Check sheet for the modelled part. Datum: model origin and axes. Units: mm. Give positions to 0.01 mm unless a question says otherwise; leave off trailing zeros. Write each loop counter-clockwise with the first axis right and the second up, starting at its lowest first coordinate (ties: lowest second). Pieces come first, ordered by that corner, then holes.
from build123d import *
from build123d.topology import SkipClean

# Parameters (mm, degrees)
SKETCH1_R           = 7.5
SKETCH1_R_2         = 4
BOSS_EXTRUDE1_DEPTH = 5
BOSS_EXTRUDE2_START = 1.1
SKETCH2_R           = 7
SKETCH2_R_2         = 4
BOSS_EXTRUDE2_DEPTH = 1.1
BOSS_EXTRUDE3_START = 32.8
SKETCH3_R           = 7.5
SKETCH3_R_2         = 4
BOSS_EXTRUDE3_DEPTH = 32.8
BOSS_EXTRUDE5_START = 1.1
SKETCH5_R           = 7
SKETCH5_R_2         = 4
BOSS_EXTRUDE5_DEPTH = 1.1
BOSS_EXTRUDE6_START = 5
SKETCH6_R           = 7.5
SKETCH6_R_2         = 4
BOSS_EXTRUDE6_DEPTH = 5


with BuildPart() as part:
    # Sketch1 → Boss-Extrude1 (new body)
    with BuildSketch(Plane(origin=(0, 0, 0), x_dir=(1, 0, 0), z_dir=(0, 1, 0))):
        with Locations(Location((0, 0, 0), (0, 0, 270))):
            Circle(SKETCH1_R)
        with Locations(Location((0, 0, 0), (0, 0, 270))):
            Circle(SKETCH1_R_2, mode=Mode.SUBTRACT)
    extrude(amount=BOSS_EXTRUDE1_DEPTH)

    # Sketch2 → Boss-Extrude2 (add)
    with SkipClean():  # the faces are left unmerged after this step: merging them gives an invalid solid
        with BuildSketch(Plane.XZ.offset(BOSS_EXTRUDE2_START)):
            with Locations(Location((0, 0, 0), (0, 0, 90))):
                Circle(SKETCH2_R)
            with Locations(Location((0, 0, 0), (0, 0, 270))):
                Circle(SKETCH2_R_2, mode=Mode.SUBTRACT)
        extrude(amount=-BOSS_EXTRUDE2_DEPTH)

    # Sketch3 → Boss-Extrude3 (add)
    with SkipClean():  # the faces are left unmerged after this step: merging them gives an invalid solid
        with BuildSketch(Plane.XZ.offset(1.1).offset(BOSS_EXTRUDE3_START)):
            with Locations(Location((0, 0, 0), (0, 0, 90))):
                Circle(SKETCH3_R)
            with Locations(Location((0, 0, 0), (0, 0, 270))):
                Circle(SKETCH3_R_2, mode=Mode.SUBTRACT)
        extrude(amount=-BOSS_EXTRUDE3_DEPTH)

    # Sketch5 → Boss-Extrude5 (add)
    with SkipClean():  # the faces are left unmerged after this step: merging them gives an invalid solid
        with BuildSketch(Plane.XZ.offset(33.9).offset(BOSS_EXTRUDE5_START)):
            with Locations(Location((0, 0, 0), (0, 0, 90))):
                Circle(SKETCH5_R)
            with Locations(Location((0, 0, 0), (0, 0, 270))):
                Circle(SKETCH5_R_2, mode=Mode.SUBTRACT)
        extrude(amount=-BOSS_EXTRUDE5_DEPTH)

    # Sketch6 → Boss-Extrude6 (add)
    with SkipClean():  # the faces are left unmerged after this step: merging them gives an invalid solid
        with BuildSketch(Plane.XZ.offset(35).offset(BOSS_EXTRUDE6_START)):
            with Locations(Location((0, 0, 0), (0, 0, 90))):
                Circle(SKETCH6_R)
            with Locations(Location((0, 0, 0), (0, 0, 270))):
                Circle(SKETCH6_R_2, mode=Mode.SUBTRACT)
        extrude(amount=-BOSS_EXTRUDE6_DEPTH)


solid = part.part
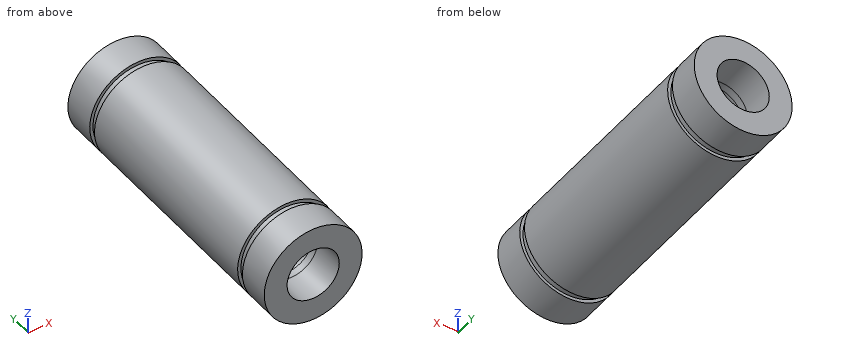
1) Sectioned sample at B-B on x = 0. Record the boundary of the cut face in (y, z), then the cut area to 3 significant figures.
2) Gauge pin test, flat ends, axial feed: pin 1 (1 mm diameter, centred on y = -30.5, z = -5.5, fed in from -X); pin 2 (5 mm diameter, centred on x = -6, y = -3.5, fed in from +Z); pin 3 (6 mm diameter, centred on x = 5.5, y = 0.5, fed in from +Z). Record the tip position at first contact, or that the pin passes through.
3) Sectioned sample at C-C on z = 5.5. Record the boundary of the cut face in (x, y).
4) Scan lines: L1, parallel to Y at x = -6.25, z = 3.5; L2, parallel to X at y = -37.15, z = 0; L3, parallel to X at y = -0.5, z = 5.75. Record each from-to range of solid material in increasing order.
5) Sectioned sample at A-A on z = 0. Record the boundary of the cut face in (x, y).
6) Sectioned sample at D-D on x = 5. Record the boundary of the cut face in (y, z).
Answers below:
1. outline: (-40, -7.5) - (-35, -7.5) - (-35, -7) - (-33.9, -7) - (-33.9, -7.5) - (-1.1, -7.5) - (-1.1, -7) - (0, -7) - (0, -7.5) - (5, -7.5) - (5, -4) - (-40, -4) - close; (-40, 4) - (5, 4) - (5, 7.5) - (0, 7.5) - (0, 7) - (-1.1, 7) - (-1.1, 7.5) - (-33.9, 7.5) - (-33.9, 7) - (-35, 7) - (-35, 7.5) - (-40, 7.5) - close
1. area: 313 mm2
2. pin 1: stops at x = -5.59
2. pin 2: stops at z = 6.63
2. pin 3: stops at z = 7.07
3. outline: (-5.1, -40) - (5.1, -40) - (5.1, -35) - (4.33, -35) - (4.33, -33.9) - (5.1, -33.9) - (5.1, -1.1) - (4.33, -1.1) - (4.33, 0) - (5.1, 0) - (5.1, 5) - (-5.1, 5) - (-5.1, 0) - (-4.33, 0) - (-4.33, -1.1) - (-5.1, -1.1) - (-5.1, -33.9) - (-4.33, -33.9) - (-4.33, -35) - (-5.1, -35) - close
4. L1: y = -40 to -35, -33.9 to -1.1, 0 to 5
4. L2: x = -7.5 to -4, 4 to 7.5
4. L3: x = -3.99 to 3.99
5. outline: (-7.5, -40) - (-4, -40) - (-4, 5) - (-7.5, 5) - (-7.5, 0) - (-7, 0) - (-7, -1.1) - (-7.5, -1.1) - (-7.5, -33.9) - (-7, -33.9) - (-7, -35) - (-7.5, -35) - close; (4, -40) - (7.5, -40) - (7.5, -35) - (7, -35) - (7, -33.9) - (7.5, -33.9) - (7.5, -1.1) - (7, -1.1) - (7, 0) - (7.5, 0) - (7.5, 5) - (4, 5) - close
6. outline: (-40, -5.59) - (-35, -5.59) - (-35, -4.9) - (-33.9, -4.9) - (-33.9, -5.59) - (-1.1, -5.59) - (-1.1, -4.9) - (0, -4.9) - (0, -5.59) - (5, -5.59) - (5, 5.59) - (0, 5.59) - (0, 4.9) - (-1.1, 4.9) - (-1.1, 5.59) - (-33.9, 5.59) - (-33.9, 4.9) - (-35, 4.9) - (-35, 5.59) - (-40, 5.59) - close
